Verification items for the finished model (mm, model axes). A direction names the side the tool comes from. Round coordinates to 2 decimals unless told otherwise and drop trailing zeros. Write each loop counter-clockwise with the first axis right and the second up, starting at its lowest first coordinate (ties: lowest second). Pieces come first, ordered by that corner, then holes. Notation, with made-up numbers: M 15.25,4 L 30.25,4 A24 ccw 30.25,25 Z; hole C 58.25,68.25 d3. An arc over 180 degrees is marked long. Answer in a Markdown table with one row per item. Add a question column.
1. Sectioned sample at C-C on y = 4. Record the cut outline in (x, z), plus the area to 3 significant figures.
2. Go/stop test with flat-tipped pins: pin 1 Ø5 at (x, z) = (0.5, -1) entering from -Y; pin 2 Ø4 at (x, z) = (2.5, -1.5) entering from +Y; pin 3 Ø0.9 at (x, y) = (-0.5, 71) entering from -Z; pin 4 Ø4 at (y, z) = (70.5, 1) entering from -X. Record where each tip stops, or that it passes through.
3. Sectioned sample at B-B on y = 98.5. Record the cut outline in (x, z).
4. Set-up check for faces 5 (the flat face through (-1.764, 60.711, -5.348)), 6 (the cylindrical face through (7.44, 94.68, 0.09)), 7 (the flat face through (-6.78, 20.33, 0.09)), 8 (the flat face through (0, 61, 4.318)): record each of +Z, -Z, +X, -X, +Y, -Y from which the full face is reachable in a straight line by a thin tool's end or side.
5. Draft check along X on faces 1 (the flat face through (1.764, 59.939, 5.348)), 2 (the cylindrical face through (-1.404, 95.277, -0.089)), 3 (the cylindrical face through (-9.305, 101.511, -4.079)), 4 (the cylindrical face through (0.223, -10.158, 0.089)). Enter one of: pulls with the +X half, pulls with the -X half, needs draft (parallel to the pull), parting line crosses it, or undercut.
6. Material ranges on probe 1 along Y at (x, z) = (-1.75, 4); probe 2 along Y at (x, z) = (5.5, 0); probe 3 along Y at (x, z) = (-4.75, 2.5), recorded low to high.
7. Sectioned sample at A-A on y = 73.5. Record the cut outline in (x, z).
8. Sectioned sample at D-D on y = 23.5. Record the cut outline in (x, z).
```python
from build123d import *

# Parameters (mm, degrees)
SKETCH1_R               = 6.477
BOSS_EXTRUDE1_DEPTH     = 6.35
CUT_EXTRUDE4_START      = 6.35
CUT_EXTRUDE4_DEPTH      = 2.032
CUT_EXTRUDE4_DRAFT      = -15
MIRROR1_START           = 6.35
MIRROR1_COPY_1_DEPTH    = 2.032
MIRROR1_COPY_1_DRAFT    = -15
CUT_EXTRUDE5_DEPTH      = 113.400381227
CUT_EXTRUDE5_DEPTH_BACK = 113.400381227
SKETCH3_OUTSIDE_W       = 47.17
SKETCH3_OUTSIDE_H       = 39.55
SKETCH3_OUTSIDE_R       = 10.16


with BuildPart() as part:
    # Sketch1 → Boss-Extrude1 (new, symmetric)
    with BuildSketch(Plane.XY):
        with BuildLine():
            Line((-10.16, 0), (-10.16, 12.7))
            Line((-10.16, 12.7), (-3.302, 28.175956627))
            Line((-3.302, 28.175956627), (-3.302, 91.991545598))
            ThreePointArc((-3.302, 91.991545598), (0, 111.76), (3.302, 91.991545598))
            Line((3.302, 91.991545598), (3.302, 28.175956627))
            Line((3.302, 28.175956627), (10.16, 12.7))
            Line((10.16, 12.7), (10.16, 0))
            ThreePointArc((10.16, 0), (0, -10.16), (-10.16, 0))
        make_face()
        Circle(SKETCH1_R, mode=Mode.SUBTRACT)
        with Locations((0, 101.6)):
            Circle(SKETCH1_R, mode=Mode.SUBTRACT)
    extrude(amount=BOSS_EXTRUDE1_DEPTH, both=True)


with BuildPart() as cut_extrude4_tool:
    # Sketch2 → Cut-Extrude4 (with draft: the straight prism first)
    with BuildSketch(Plane.XY.offset(CUT_EXTRUDE4_START)):
        with BuildLine():
            ThreePointArc((0.508, 31.242), (1.585630735, 31.688369265), (2.032, 32.766))
            Line((2.032, 32.766), (2.032, 87.884))
            ThreePointArc((2.032, 87.884), (1.585630735, 88.961630735), (0.508, 89.408))
            Line((0.508, 89.408), (-0.508, 89.408))
            ThreePointArc((-0.508, 89.408), (-1.585630735, 88.961630735), (-2.032, 87.884))
            Line((-2.032, 87.884), (-2.032, 32.766))
            ThreePointArc((-2.032, 32.766), (-1.585630735, 31.688369265), (-0.508, 31.242))
            Line((-0.508, 31.242), (0.508, 31.242))
        make_face()
    extrude(amount=-CUT_EXTRUDE4_DEPTH)
    # Cut-Extrude4: the draft: its side faces are tilted about the plane it starts from
    cut_extrude4_sides = [cut_extrude4_tool.faces().sort_by_distance(p)[0] for p in [
        (-1.585630735, 31.688369265, 5.334),
        (0, 31.242, 5.334),
        (1.585630735, 31.688369265, 5.334),
        (2.032, 60.325, 5.334),
        (1.585630735, 88.961630735, 5.334),
        (0, 89.408, 5.334),
        (-1.585630735, 88.961630735, 5.334),
        (-2.032, 60.325, 5.334),
    ]]
    draft(cut_extrude4_sides, Plane.XY.offset(CUT_EXTRUDE4_START), CUT_EXTRUDE4_DRAFT)


with BuildPart() as part_1:
    add(part.part)

    # Cut-Extrude4: cut by cut_extrude4_tool
    add(cut_extrude4_tool.part, mode=Mode.SUBTRACT)


with BuildPart() as mirror1_copy_1_tool:
    # Mirror1 copy 1 sketch → Mirror1 copy 1 (with draft: the straight prism first)
    with BuildSketch(Plane(origin=(0, 0, 0), x_dir=(1, 0, 0), z_dir=(0, 0, -1)).offset(MIRROR1_START)):
        with BuildLine():
            ThreePointArc((0.508, -31.242), (1.585630735, -31.688369265), (2.032, -32.766))
            Line((2.032, -32.766), (2.032, -87.884))
            ThreePointArc((2.032, -87.884), (1.585630735, -88.961630735), (0.508, -89.408))
            Line((0.508, -89.408), (-0.508, -89.408))
            ThreePointArc((-0.508, -89.408), (-1.585630735, -88.961630735), (-2.032, -87.884))
            Line((-2.032, -87.884), (-2.032, -32.766))
            ThreePointArc((-2.032, -32.766), (-1.585630735, -31.688369265), (-0.508, -31.242))
            Line((-0.508, -31.242), (0.508, -31.242))
        make_face()
    extrude(amount=-MIRROR1_COPY_1_DEPTH)
    # Mirror1 copy 1: the draft: its side faces are tilted about the plane it starts from
    mirror1_copy_1_sides = [mirror1_copy_1_tool.faces().sort_by_distance(p)[0] for p in [
        (-1.585630735, 31.688369265, -5.334),
        (0, 31.242, -5.334),
        (1.585630735, 31.688369265, -5.334),
        (2.032, 60.325, -5.334),
        (1.585630735, 88.961630735, -5.334),
        (0, 89.408, -5.334),
        (-1.585630735, 88.961630735, -5.334),
        (-2.032, 60.325, -5.334),
    ]]
    draft(mirror1_copy_1_sides, Plane(origin=(0, 0, 0), x_dir=(1, 0, 0), z_dir=(0, 0, -1)).offset(MIRROR1_START), MIRROR1_COPY_1_DRAFT)


with BuildPart() as part_2:
    add(part_1.part)

    # Mirror1 copy 1: cut by mirror1_copy_1_tool
    add(mirror1_copy_1_tool.part, mode=Mode.SUBTRACT)

    # Sketch3 outside → Cut-Extrude5 (cut, two sides: drawn at the far end of the back side and taken through both)
    with BuildSketch(Plane(origin=(0, 0, 0), x_dir=(1, 0, 0), z_dir=(0, 1, 0)).offset(-CUT_EXTRUDE5_DEPTH_BACK)):
        Rectangle(SKETCH3_OUTSIDE_W, SKETCH3_OUTSIDE_H)
        Circle(SKETCH3_OUTSIDE_R, mode=Mode.SUBTRACT)
    extrude(amount=CUT_EXTRUDE5_DEPTH + CUT_EXTRUDE5_DEPTH_BACK, mode=Mode.SUBTRACT)


solid = part_2.part
```
Geometry check:
| question | item | result |
|---|---|---|
| 1 | outline | M -7.93,-6.35 L -5.09,-6.35 L -5.09,6.35 L -7.93,6.35 A10.16 ccw Z; M 5.09,-6.35 L 7.93,-6.35 A10.16 ccw 7.93,6.35 L 5.09,6.35 Z |
| 1 | area | 111 mm2 |
| 2 | pin 1 | stops at y = -10.16 |
| 2 | pin 2 | stops at y = 111.75 |
| 2 | pin 3 | stops at z = -4.32 |
| 2 | pin 4 | stops at x = -3.3 |
| 3 | outline | M -9.68,-3.1 A10.16 ccw -7.93,-6.35 L -5.69,-6.35 L -5.69,6.35 L -7.93,6.35 A10.16 ccw -9.68,3.1 Z; M 5.69,-6.35 L 7.93,-6.35 A10.16 ccw 9.68,-3.1 L 9.68,3.1 A10.16 ccw 7.93,6.35 L 5.69,6.35 Z |
| 4 | face 5 | -Z |
| 4 | face 6 | +Z, -Z, +X |
| 4 | face 7 | +Z, -Z, -X |
| 4 | face 8 | +Z |
| 5 | face 1 | undercut |
| 5 | face 2 | undercut |
| 5 | face 3 | pulls with the -X half |
| 5 | face 4 | parting line crosses it |
| 6 | probe 1 | y = -10.01 to -6.24, 6.24 to 95.36, 107.84 to 111.61 |
| 6 | probe 2 | y = -8.54 to -3.42, 3.42 to 23.22, 93.06 to 98.18, 105.02 to 110.14 |
| 6 | probe 3 | y = -8.98 to -4.4, 4.4 to 24.91, 92.62 to 97.2, 106 to 110.58 |
| 7 | outline | M -3.3,-6.35 L -2.03,-6.35 L -1.49,-4.32 L 1.49,-4.32 L 2.03,-6.35 L 3.3,-6.35 L 3.3,6.35 L 2.03,6.35 L 1.49,4.32 L -1.49,4.32 L -2.03,6.35 L -3.3,6.35 Z |
| 8 | outline | M -5.37,-6.35 L 5.37,-6.35 L 5.37,6.35 L -5.37,6.35 Z |
